Build history of the part. All positions in model axes, mm. A direction names the side the tool comes from. Give positions to 0.01 mm unless a question says otherwise; leave off trailing zeros. Order: outer loops, then holes, each group sorted by start corner. A loop starts at its lowest first (then second) coordinate and runs counter-clockwise, first axis right, second up. Notation, with made-up numbers: (-1, 12) - (12, 12) arc R13 ccw to (12, 37) - close; hole circle Ø3 at (-36.75, 6). An arc over 180 degrees is marked (long way). One line per item, written item: value.
Autodesk Inventor part; units mm, degrees
ref_plane "YZ Plane" through (0, 0, 0) normal (1, 0, 0) x (0, 1, 0)
ref_plane "XZ Plane" through (0, 0, 0) normal (0, 1, 0) x (-1, 0, 0)
ref_plane "XY Plane" through (0, 0, 0) normal (0, 0, 1) x (1, 0, 0)
sketch "Sketch1" plane through (0, 0, 0) normal (0, 1, 0) x (-1, 0, 0)
  line L0 (30, 29) -> (-30, 29)
  line L1 (-30, 29) -> (-30, -29)
  line L2 (-30, -29) -> (30, -29)
  line L3 (30, -29) -> (30, 29)
  line L4 (30, 29) -> (-30, -29) construction
  line L5 (-30, 29) -> (30, -29) construction
  point P0 (0, 0)
  dimension "d0" = 60
  dimension "d1" = 58
extrude "Extrusion1" add sketch "Sketch1" along normal blind 15
sketch "Sketch2" plane through (0, 15, 0) normal (0, 1, 0) x (1, 0, 0)
  line L0 (30, -29) -> (30, 29)
  line L1 (30, 29) -> (-30, 29)
  line L2 (-30, 29) -> (-30, -29)
  line L3 (-30, -29) -> (30, -29)
  line L4 (-30, 0) -> (30, 0) construction
  point P0 (0, 0)
  point P1 (-15, -15)
  point P2 (-15, 15)
  point P3 (0, 0)
  point P4 (12, -5)
  dimension "d4" = 30
  dimension "d5" = 15
  dimension "d22" = 12
  dimension "d23" = 5
hole "Hole1" at (12, 15, 5) direction (0, -1, 0) diameter 10.106 end through all
hole "Hole2" at (-15, 15, 15) at (-15, 15, -15) direction (0, -1, 0) diameter 6 end through all counterbore diameter 11 counterbore depth 7
properties part number "Lift Bracket"
(1) Slice it at A-A, the plane z = -15. Give the cut face in (x, y).
Completed:
outline: (-30, 0) - (-18, 0) - (-18, 8) - (-20.5, 8) - (-20.5, 15) - (-30, 15) - close; (-12, 0) - (30, 0) - (30, 15) - (-9.5, 15) - (-9.5, 8) - (-12, 8) - close
(2) Slice it at C-C, the plane x = 12. Give the cut face in (y, z).
Completed:
outline: (0, -29) - (15, -29) - (15, -0.05) - (0, -0.05) - close; (0, 10.05) - (15, 10.05) - (15, 29) - (0, 29) - close
(3) Drill centre lines: line 1 (Z direction, x = -15, y = 4.5); line 2 (X direction, y = 6.25, z = 15); line 3 (Z direction, x = 12, y = 11). Where is each one in solid material? Low to high.
Completed:
line 1: -29 to -18, -12 to 12, 18 to 29
line 2: -30 to -18, -12 to 30
line 3: -29 to -0.05, 10.05 to 29
(4) Slice it at B-B, the plane x = -15. Give the cut face in (y, z).
Completed:
outline: (0, -29) - (15, -29) - (15, -20.5) - (8, -20.5) - (8, -18) - (0, -18) - close; (0, -12) - (8, -12) - (8, -9.5) - (15, -9.5) - (15, 9.5) - (8, 9.5) - (8, 12) - (0, 12) - close; (0, 18) - (8, 18) - (8, 20.5) - (15, 20.5) - (15, 29) - (0, 29) - close
(5) Pull direction Z, two halves, no side cores. Call faces 1 (the face through (30, 7, 0)), 2 (the face through (0, 7, 29)), 3 (the face through (-12.6, 8, -12.6)), 4 (the face through (-9.63, 11.45, -16.19)): +Z half, -Z half, draft (parallel to the pull), parting line (faces both ways), or undercut.
Completed:
face 1: draft
face 2: +Z half
face 3: undercut
face 4: undercut
(6) 3-axis set-ups, long thin cutter, end or side, ignore diameter. For faces 5 (the face through (-12.6, 8, 17.4)), 6 (the face through (-30, 7, 0)): which of +Z, -Z, +X, -X, +Y, -Y reach the whole face in a straight line?
Completed:
face 5: +Y
face 6: +Z, -Z, -X, +Y, -Y
(7) Pin check, flat tips, straight feed: P1, Ø5.5, axis at x = -15.5, z = -17, coming from the +Y side; P2, Ø3.5, axis at x = -15, z = -15, coming from the -Y side. Stop position of each tip, or through.
Completed:
P1: y = 8
P2: through
(8) Slice it at D-D, the plane y = 9.75. Give the cut face in (x, z).
Completed:
outline: (-30, -29) - (30, -29) - (30, 29) - (-30, 29) - close; hole circle Ø11 at (-15, -15); hole circle Ø11 at (-15, 15); hole circle Ø10.11 at (12, 5)
